The listing builds one solid part. Answer for the finished solid, in the listing's coordinates (mm). A direction names the side the tool comes from. Give positions to 0.01 mm unless a question says otherwise; leave off trailing zeros. Loops run counter-clockwise (first coordinate to the right, second up) from the corner with the lowest first, then second, coordinate; pieces in that order, holes last. Notation, with made-up numbers: M 27.5,22.5 L 32.5,22.5 A33 cw 32.5,53.5 Z; hole C -25.5,-17.5 d1. An arc over 180 degrees is marked long. Return JSON: item names as keys, results as strings.
from build123d import *

# Parameters (mm, degrees)
F0_W          = 6.4
F0_H          = 3.175
F2_S5_R       = 6.4
F2_T6_DEPTH   = 14
F3_R          = 4.85
F4_DEPTH      = 25
F4_DEPTH_BACK = 25


# Not quite as in the source:
# - a fillet or chamfer that OpenCascade refuses, or shapes differently, is made with other operations: its cross-section is extruded or revolved along the edge and cut away or added


with BuildPart() as f1:
    # F0 (on Front) → F1 (revolve)
    with BuildSketch(Plane.XZ):
        with Locations((3.2, 0)):
            Rectangle(F0_W, F0_H)
        Polygon((0, 1.5875), (6.4, 1.5875), (9, 1.5875), (9, 11.5875), (0, 11.5875), align=None)
    revolve(axis=Axis((0, 0, 6.5875), (0, 0, -1)))

    # F2: chamfer of 3 on 1 edges, made by hand


with BuildPart() as f2_tool2:
    # F2_s3 → F2_t4 (revolve)
    with BuildSketch(Plane.XZ):
        Polygon((6, 1.5875), (9, 4.5875), (9, 1.5875), align=None)
    revolve(axis=Axis((0, 0, 1.5875), (0, 0, -1)))

    # F2_s5 → F2_t6 (cut, symmetric)
    with BuildSketch(Plane.XY.offset(3.1)):
        Circle(F2_S5_R)
    extrude(amount=F2_T6_DEPTH, both=True, mode=Mode.SUBTRACT)


with BuildPart() as f1_1:
    add(f1.part)

    # F2_t1: cut F2_tool2
    add(f2_tool2.part, mode=Mode.SUBTRACT)

    # F3 (on Top) → F4 (cut, two sides)
    with BuildSketch(Plane.XY) as f4_sk:
        with Locations((-1.1, 0)):
            Circle(F3_R)
    extrude(amount=-F4_DEPTH, mode=Mode.SUBTRACT)
    extrude(f4_sk.sketch, amount=F4_DEPTH_BACK, mode=Mode.SUBTRACT)


solid = f1_1.part
(1) The part is cut by section B-B (x = 0). Determine the outline of the cut face in (y, z).
Values follow:
{"outline": "M -9,4.59 L -6.4,1.99 L -6.4,-1.59 L -4.72,-1.59 L -4.72,11.59 L -9,11.59 Z; M 4.72,-1.59 L 6.4,-1.59 L 6.4,1.99 L 9,4.59 L 9,11.59 L 4.72,11.59 Z"}
(2) Given pin 1 (6 mm diameter, centred on x = 4.5, z = 9.5, fed in from +Y); pin 2 (3 mm diameter, centred on y = 6.5, z = 3, fed in from +X); pin 3 (3 mm diameter, centred on x = -3.5, z = 0, fed in from +Y); pin 4 (3 mm diameter, centred on x = -2.5, y = 2.5, fed in from +Z), each flat-ended and moving along its own axis, determine where each tip first touches the part or whether it passes through.
Values follow:
{"pin 1": "y = 8.87", "pin 2": "x = 6.55", "pin 3": "y = 6.08", "pin 4": "through"}
(3) Straight lines are drawn through the part: line 1 along X through (y, z) = (0, 6); line 2 along Y through (x, z) = (-2.25, 11.25); line 3 along Y through (x, z) = (-1.1, 3). For each, find the intervals that lie inside material, in ascending order.
Values follow:
{"line 1": "-9 to -5.95, 3.75 to 9", "line 2": "-8.71 to -4.71, 4.71 to 8.71", "line 3": "-7.33 to -4.85, 4.85 to 7.33"}
(4) The part is cut by section C-C (z = 0.75). Determine the outline of the cut face in (x, y), and give its area (3 significant figures).
Values follow:
{"outline": "C 0,0 d12.8; hole C -1.1,0 d9.7", "area": "54.8 mm²"}
(5) The part is cut by section A-A (y = 0). Determine the outline of the cut face in (x, z).
Values follow:
{"outline": "M -9,4.59 L -6.4,1.99 L -6.4,-1.59 L -5.95,-1.59 L -5.95,11.59 L -9,11.59 Z; M 3.75,-1.59 L 6.4,-1.59 L 6.4,1.99 L 9,4.59 L 9,11.59 L 3.75,11.59 Z"}
(6) The part is cut by section D-D (z = 6.25). Determine the outline of the cut face in (x, y).
Values follow:
{"outline": "C 0,0 d18; hole C -1.1,0 d9.7"}
(7) A tool of negligible diameter and unlimited length cuts with its end or side. For faces 1 (the cylindrical face through (-1.172, -8.923, 8.136)), 2 (the cylindrical face through (-5.08, 3.89, 0.23)), from which of +Z, -Z, +X, -X, +Y, -Y can it reach the whole face along a straight path? Write none if from no direction.
Values follow:
{"face 1": "+Z, -Z", "face 2": "-Z"}
